from build123d import *

# Parameters (mm, degrees)
BOSS_EXTRUDE1_DEPTH             = 36.158
TAP_DRILL_FOR_M3X0_5_TAP1_D     = 2.5
TAP_DRILL_FOR_M3X0_5_TAP1_DEPTH = 12.7
TAP_DRILL_FOR_M3X0_5_TAP1_TIP   = 0.751075774
SKETCH4_R                       = 11
BOSS_EXTRUDE2_DEPTH             = 2
SKETCH5_R                       = 2.5
BOSS_EXTRUDE3_DEPTH             = 22
CUT_EXTRUDE1_DEPTH              = 19.558


with BuildPart() as part:
    # Sketch1 → Boss-Extrude1 (new body)
    with BuildSketch(Plane(origin=(0, 0, 0), x_dir=(1, 0, 0), z_dir=(0, 1, 0))):
        Polygon((-21.15, 16.07), (-16.07, 21.15), (16.07, 21.15), (21.15, 16.07), (21.15, -16.07), (16.07, -21.15), (-16.07, -21.15), (-21.15, -16.07), align=None)
    extrude(amount=BOSS_EXTRUDE1_DEPTH)

    # Tap Drill for M3x0.5 Tap1
    with Locations(Plane(origin=(0, 36.158, 0), x_dir=(1, 0, 0), z_dir=(0, 1, 0))):
        with Locations((-15.5, 15.5), (15.5, 15.5), (15.5, -15.5), (-15.5, -15.5)):
            Hole(TAP_DRILL_FOR_M3X0_5_TAP1_D / 2, depth=TAP_DRILL_FOR_M3X0_5_TAP1_DEPTH)
            with Locations((0, 0, -(TAP_DRILL_FOR_M3X0_5_TAP1_DEPTH + TAP_DRILL_FOR_M3X0_5_TAP1_TIP / 2))):  # 118° drill point
                Cone(0, TAP_DRILL_FOR_M3X0_5_TAP1_D / 2, TAP_DRILL_FOR_M3X0_5_TAP1_TIP, mode=Mode.SUBTRACT)

    # Sketch4 → Boss-Extrude2 (add)
    with BuildSketch(Plane(origin=(0, 36.158, 0), x_dir=(1, 0, 0), z_dir=(0, 1, 0))):
        Circle(SKETCH4_R)
    extrude(amount=BOSS_EXTRUDE2_DEPTH)

    # Sketch5 → Boss-Extrude3 (add)
    with BuildSketch(Plane(origin=(0, 38.158, 0), x_dir=(1, 0, 0), z_dir=(0, 1, 0))):
        Circle(SKETCH5_R)
    extrude(amount=BOSS_EXTRUDE3_DEPTH)

    # Sketch6 → Cut-Extrude1 (cut)
    with BuildSketch(Plane(origin=(0, 60.158, 0), x_dir=(1, 0, 0), z_dir=(0, 1, 0))):
        with BuildLine():
            Line((1.623373896, 1.901225182), (1.623373896, -1.901225182))
            ThreePointArc((1.623373896, -1.901225182), (2.5, 0), (1.623373896, 1.901225182))
        make_face()
    extrude(amount=-CUT_EXTRUDE1_DEPTH, mode=Mode.SUBTRACT)


solid = part.part
Geometry check sheet. Reference: the model listing, model coordinates, mm. A direction names the side the tool comes from. Give positions to 0.01 mm unless a question says otherwise; leave off trailing zeros. Order: outer loops, then holes, each group sorted by start corner. A loop starts at its lowest first (then second) coordinate and runs counter-clockwise, first axis right, second up. Notation, with made-up numbers: (25, -24.75) - (50, -24.75) arc R22 cw to (50, 6.25) - close; hole circle Ø3 at (17.25, 29). An arc over 180 degrees is marked (long way). Answer as a JSON object with one key per item and string values.
(1) Tool access check on faces 5 (the flat face through (-9, 36.158, 9)), 6 (the flat face through (1.623, 51, 0)), 7 (the flat face through (0, 0, 0)). Record the directions out of +Z, -Z, +X, -X, +Y, -Y that give a thin tool (end or side, any length) a straight path to the whole face; none if there is none.
Report:
{"face 5": "+Y", "face 6": "+Z, -Z, +X, +Y", "face 7": "+Z, -Z, +X, -X, -Y"}
(2) Cross-section at A-A (x = 0). Record the cut outline in (y, z).
Report:
{"outline": "(0, -21.15) - (36.16, -21.15) - (36.16, -11) - (38.16, -11) - (38.16, -2.5) - (60.16, -2.5) - (60.16, 2.5) - (38.16, 2.5) - (38.16, 11) - (36.16, 11) - (36.16, 21.15) - (0, 21.15) - close"}
(3) Cross-section at B-B (y = 17). Record the cut outline in (x, z).
Report:
{"outline": "(-21.15, -16.07) - (-16.07, -21.15) - (16.07, -21.15) - (21.15, -16.07) - (21.15, 16.07) - (16.07, 21.15) - (-16.07, 21.15) - (-21.15, 16.07) - close"}
(4) Cross-section at D-D (y = 51.5). Record the cut outline in (x, z), then the cut area to 3 significant figures.
Report:
{"outline": "(1.62, -1.9) - (1.62, 1.9) arc R2.5 ccw (long way) to start", "area": "17.3 mm^2"}
(5) Depth check by flat-ended pin: pin 1 Ø1.5 at (x, z) = (12.5, 9.5) entering from +Y; pin 2 Ø5 at (x, y) = (-2, 43) entering from +Z; pin 3 Ø1.9 at (y, z) = (50, 1) entering from +X. Enter the tip coordinate at first touch or a pass-through.
Report:
{"pin 1": "y = 36.16", "pin 2": "z = 2.5", "pin 3": "x = 1.62"}
(6) Draft check along Z on faces 1 (the flat face through (-3, 38.158, 0)), 2 (the cylindrical face through (-14.579, 29.719, -16.345)), 3 (the flat face through (18.57, 17.83, -18.65)), 4 (the flat face through (18.65, 17.83, 18.57)). Enter one of: released by +Z, released by -Z, zero draft, split by the parting line, or undercut.
Report:
{"face 1": "zero draft", "face 2": "undercut", "face 3": "released by -Z", "face 4": "released by +Z"}
(7) Material ranges on line 1 (Z direction, x = 15.5, y = 32.5); line 2 (Z direction, x = -15, y = 31), recorded low to high.
Report:
{"line 1": "-21.15 to -16.75, -14.25 to 14.25, 16.75 to 21.15", "line 2": "-21.15 to -16.65, -14.35 to 14.35, 16.65 to 21.15"}
(8) Cross-section at C-C (z = 9.5). Record the cut outline in (x, y), then the cut area to 3 significant figures.
Report:
{"outline": "(-21.15, 0) - (21.15, 0) - (21.15, 36.16) - (5.55, 36.16) - (5.55, 38.16) - (-5.55, 38.16) - (-5.55, 36.16) - (-21.15, 36.16) - close", "area": "1,550 mm^2"}
